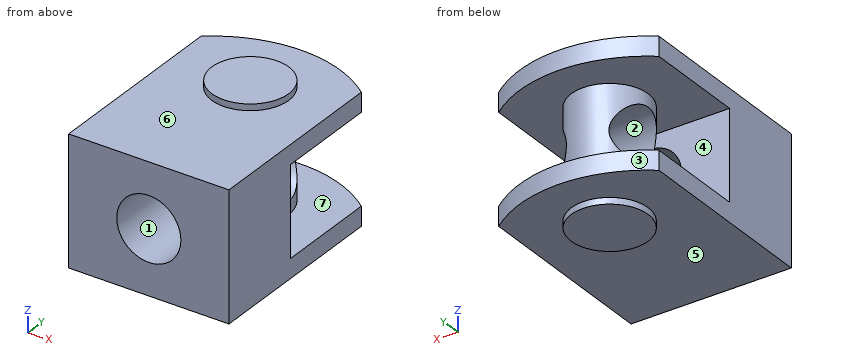
from build123d import *

# Parameters (mm, degrees)
SKETCH1_R                = 5
BOSS_EXTRUDE1_DEPTH      = 10
CUT_EXTRUDE1_DEPTH       = 34.179441681
CUT_EXTRUDE1_DEPTH_BACK  = 34.179441681
BOSS_EXTRUDE2_DEPTH      = 1
BOSS_EXTRUDE2_DEPTH_BACK = 21
SKETCH4_R                = 6
SKETCH5_R                = 5
CUT_EXTRUDE3_DEPTH       = 7.5
SKETCH6_R                = 5
CUT_EXTRUDE4_DEPTH       = 15


with BuildPart() as part:
    # Sketch1 → Boss-Extrude1 (new, symmetric)
    with BuildSketch(Plane.XY):
        with BuildLine():
            Line((-12.5, 15), (-12.5, -15))
            Line((-12.5, -15), (12.5, -15))
            Line((12.5, -15), (12.5, 15))
            ThreePointArc((12.5, 15), (0, 19.387505004), (-12.5, 15))
        make_face()
        with Locations((0, 8)):
            Circle(SKETCH1_R, mode=Mode.SUBTRACT)
    extrude(amount=BOSS_EXTRUDE1_DEPTH, both=True)

    # Sketch2 → Cut-Extrude1 (cut, two sides: drawn at the far end of the back side and taken through both)
    with BuildSketch(Plane(origin=(12.5, 0, 0), x_dir=(0, 0, -1), z_dir=(1, 0, 0)).offset(-CUT_EXTRUDE1_DEPTH_BACK)):
        Polygon((0, -1), (-7, -1), (-7, 28.013491334), (7, 28.013491334), (7, -1), align=None)
    extrude(amount=CUT_EXTRUDE1_DEPTH + CUT_EXTRUDE1_DEPTH_BACK, mode=Mode.SUBTRACT)

    # Sketch4 → Boss-Extrude2 (add, two sides: drawn at the far end of the back side and taken through both)
    with BuildSketch(Plane.XY.offset(10).offset(-BOSS_EXTRUDE2_DEPTH_BACK)):
        with Locations((0, 8)):
            Circle(SKETCH4_R)
    extrude(amount=BOSS_EXTRUDE2_DEPTH + BOSS_EXTRUDE2_DEPTH_BACK)

    # Sketch5 → Cut-Extrude3 (cut, symmetric)
    with BuildSketch(Plane(origin=(0, 0, 0), x_dir=(0, 0, -1), z_dir=(1, 0, 0))):
        with Locations((0, 8)):
            Circle(SKETCH5_R)
    extrude(amount=CUT_EXTRUDE3_DEPTH, both=True, mode=Mode.SUBTRACT)

    # Sketch6 → Cut-Extrude4 (cut)
    with BuildSketch(Plane.XZ.offset(15)):
        with Locations(Location((0, 0, 0), (0, 0, 270))):
            Circle(SKETCH6_R)
    extrude(amount=-CUT_EXTRUDE4_DEPTH, mode=Mode.SUBTRACT)


solid = part.part
Read the model definition and answer for the solid it produces. Units are mm, in the model's axes. Face numbers are marked on the shaded views. A direction names the side the tool comes from. Give positions to 0.01 mm unless a question says otherwise; leave off trailing zeros. Write each loop counter-clockwise with the first axis right and the second up, starting at its lowest first coordinate (ties: lowest second). Pieces come first, ordered by that corner, then holes. Notation, with made-up numbers: (-36.5, 57.5) - (-28.5, 57.5) arc R12 ccw to (-28.5, 78.5) - close; hole circle Ø5 at (-23.5, 44.5). An arc over 180 degrees is marked (long way). Answer in a Markdown table with one row per item. Add a question column.
Item 1: Section C-C, the plane x = 0 is taken. Write down the section's boundary in (y, z).
Item 2: Flat-ended cylindrical pins translate along their axes: P1, Ø8, axis at x = 0, z = 0, coming from the +Y side; P2, Ø4, axis at x = -5.5, y = -9.5, coming from the +Z side; P3, Ø2, axis at x = 0, y = -3.5, coming from the -Z side. Find the tip coordinate at first contact, or state that the pin passes through.
Item 3: Determine the mould class of the marked faces 1, 2 and 3 for opening direction X: pulls with the +X half, pulls with the -X half, needs draft (parallel to the pull), parting line crosses it, or undercut.
Item 4: Section D-D, the plane x = -3.75 is taken. Write down the section's boundary in (y, z).
Item 5: Section B-B, the plane z = 3.75 is taken. Write down the section's boundary in (x, y), and give its area (3 significant figures).
Item 6: Section A-A, the plane y = 8 is taken. Write down the section's boundary in (x, z).
Item 7: A tool of negligible diameter and unlimited length cuts with its end or side. For the marked faces 4, 5, 6 and 7, from which of +Z, -Z, +X, -X, +Y, -Y can it reach the whole face along a straight path? Write none if from no direction.
Item 8: Find the intervals of material crossed by L1, parallel to Z at x = 2, y = 8; L2, parallel to Z at x = 6.25, y = 13.5; L3, parallel to X at y = -7, z = 0, in increasing order.
Recorded:
| question | item | result |
|---|---|---|
| 1 | outline | (-15, -10) - (2, -10) - (2, -11) - (14, -11) - (14, -10) - (19.39, -10) - (19.39, -7) - (14, -7) - (14, 7) - (19.39, 7) - (19.39, 10) - (14, 10) - (14, 11) - (2, 11) - (2, 10) - (-15, 10) - (-15, 5) - (-1, 5) - (-1, 7) - (2, 7) - (2, -7) - (-1, -7) - (-1, -5) - (-15, -5) - close; hole circle Ø10 at (8, 0) |
| 2 | P1 | stops at y = 14 |
| 2 | P2 | stops at z = 10 |
| 2 | P3 | stops at z = -10 |
| 3 | face 1 | undercut |
| 3 | face 2 | needs draft |
| 3 | face 3 | parting line crosses it |
| 4 | outline | (-15, -10) - (3.32, -10) - (3.32, -11) - (12.68, -11) - (12.68, -10) - (19.03, -10) - (19.03, -7) - (12.68, -7) - (12.68, -1.75) arc R5 cw to (3.32, -1.75) - (3.32, -7) - (-1, -7) - (-1, -3.31) - (-15, -3.31) - close; (-15, 3.31) - (-1, 3.31) - (-1, 7) - (3.32, 7) - (3.32, 1.75) arc R5 cw to (12.68, 1.75) - (12.68, 7) - (19.03, 7) - (19.03, 10) - (12.68, 10) - (12.68, 11) - (3.32, 11) - (3.32, 10) - (-15, 10) - close |
| 5 | outline | (-12.5, -15) - (-3.31, -15) - (-3.31, -1) - (-12.5, -1) - close; (-5.01, 4.69) arc R6 ccw to (5.01, 4.69) - close; (-5.01, 11.31) - (5.01, 11.31) arc R6 ccw to start; (3.31, -15) - (12.5, -15) - (12.5, -1) - (3.31, -1) - close |
| 5 | area | 295 mm2 |
| 6 | outline | (-12.5, -10) - (-6, -10) - (-6, -11) - (6, -11) - (6, -10) - (12.5, -10) - (12.5, -7) - (6, -7) - (6, -5) - (-6, -5) - (-6, -7) - (-12.5, -7) - close; (-12.5, 7) - (-6, 7) - (-6, 5) - (6, 5) - (6, 7) - (12.5, 7) - (12.5, 10) - (6, 10) - (6, 11) - (-6, 11) - (-6, 10) - (-12.5, 10) - close |
| 7 | face 4 | +X, -X |
| 7 | face 5 | -Z |
| 7 | face 6 | +Z |
| 7 | face 7 | none |
| 8 | L1 | z = -11 to -5, 5 to 11 |
| 8 | L2 | z = -10 to -7, 7 to 10 |
| 8 | L3 | x = -12.5 to -5, 5 to 12.5 |
